Source: CAD feature listing. Evaluate the final solid. Frame: model axes, mm. Face numbers are marked on the shaded views. A direction names the side the tool comes from. Give positions to 0.01 mm unless a question says otherwise; leave off trailing zeros. Loops run counter-clockwise (first coordinate to the right, second up) from the corner with the lowest first, then second, coordinate; pieces in that order, holes last. Notation, with made-up numbers: M -32,21.25 L 24,21.25 A22 cw 24,40.25 Z; hole C -20,43.5 d11. An arc over 180 degrees is marked long. Answer in a Markdown table with one row per item.
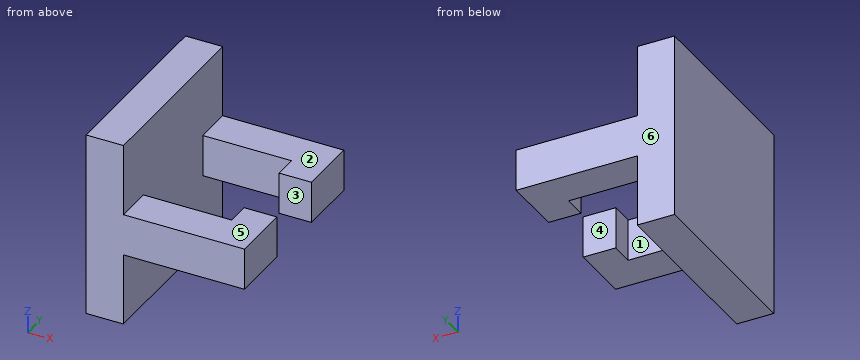
```python
from build123d import *

# Parameters (mm, degrees)
F0_W     = 40
F0_H     = 40
F1_DEPTH = 40
F4_DEPTH = 40
F3_W     = 32
F3_H     = 15.5
F5_DEPTH = 40
F6_DEPTH = 40


with BuildPart() as f1:
    # F0 (on Top) → F1 (new body)
    with BuildSketch(Plane.XY):
        Rectangle(F0_W, F0_H)
    extrude(amount=-F1_DEPTH)

    # F2 (on face) → F4 (cut)
    with BuildSketch(Plane.XY):
        Polygon((20, 20), (14.041499, 20), (14.041499, 7), (7.041499, 7), (7.041499, 12), (-12, 12), (-12, -12), (7.041499, -12), (7.041499, -7), (14.041499, -7), (14.041499, -20), (20, -20), align=None)
    extrude(amount=-F4_DEPTH, mode=Mode.SUBTRACT)

    # F3 (on face) → F5 (cut)
    with BuildSketch(Plane.XZ.offset(20)):
        with Locations((4, -7.75)):
            Rectangle(F3_W, F3_H)
    extrude(amount=-F5_DEPTH, mode=Mode.SUBTRACT)

    # F3 (on face) → F6 (cut)
    with BuildSketch(Plane.XZ.offset(20)):
        with Locations((4, -32.25)):
            Rectangle(F3_W, F3_H)
    extrude(amount=-F6_DEPTH, mode=Mode.SUBTRACT)


solid = f1.part
```
1) Pin query (flat end, axial travel): pin 1 Ø12 at (y, z) = (-6.5, -33) entering from +X; pin 2 Ø12 at (x, z) = (-10, -15) entering from +Y; pin 3 Ø10.5 at (x, y) = (2, 16.5) entering from +Z; pin 4 Ø5 at (x, y) = (7.5, 8) entering from -Z. Return the tip coordinate at first contact, or that it passes through.
Reply:
| item | result |
|---|---|
| pin 1 | stops at x = -12 |
| pin 2 | stops at y = 20 |
| pin 3 | stops at z = -15.5 |
| pin 4 | stops at z = -24.5 |
2) Pull-direction query (Y, two-part tool) for the marked faces 4, 5 and 6; classes: released by +Y, released by -Y, zero draft, split by the parting line, or undercut.
Reply:
| item | result |
|---|---|
| face 4 | undercut |
| face 5 | zero draft |
| face 6 | released by +Y |
3) Section A-A, the plane x = 3. Return loops of the section in (y, z), then the cut area to 3 significant figures.
Reply:
| item | result |
|---|---|
| outline | M -20,-24.5 L -12,-24.5 L -12,-15.5 L -20,-15.5 Z; M 12,-24.5 L 20,-24.5 L 20,-15.5 L 12,-15.5 Z |
| area | 144 mm² |
4) Section B-B, the plane y = -8.5. Return loops of the section in (x, z), then the cut area to 3 significant figures.
Reply:
| item | result |
|---|---|
| outline | M -20,-40 L -12,-40 L -12,0 L -20,0 Z; M 7.04,-24.5 L 14.04,-24.5 L 14.04,-15.5 L 7.04,-15.5 Z |
| area | 383 mm² |
5) Section C-C, the plane z = -22.5. Return loops of the section in (x, y).
Reply:
| item | result |
|---|---|
| outline | M -20,-20 L 14.04,-20 L 14.04,-7 L 7.04,-7 L 7.04,-12 L -12,-12 L -12,12 L 7.04,12 L 7.04,7 L 14.04,7 L 14.04,20 L -20,20 Z |
6) Set-up query: the marked faces 1, 2 and 3. Return all of +Z, -Z, +X, -X, +Y, -Y with unobstructed straight access to the full face (end or side cutting, diameter ignored); none if empty.
Reply:
| item | result |
|---|---|
| face 1 | +Z, -Z |
| face 2 | +Z, +X, +Y, -Y |
| face 3 | +Z, -Z, +X |
7) Material intervals for L1, parallel to Y at x = -3, z = -16; L2, parallel to Z at x = -5, y = 16.5; L3, parallel to X at y = 1.5, z = -36.5, sorted ascending.
Reply:
| item | result |
|---|---|
| L1 | y = -20 to -12, 12 to 20 |
| L2 | z = -24.5 to -15.5 |
| L3 | x = -20 to -12 |
8) Section D-D, the plane y = 13. Return loops of the section in (x, z).
Reply:
| item | result |
|---|---|
| outline | M -20,-40 L -12,-40 L -12,-24.5 L 14.04,-24.5 L 14.04,-15.5 L -12,-15.5 L -12,0 L -20,0 Z |
